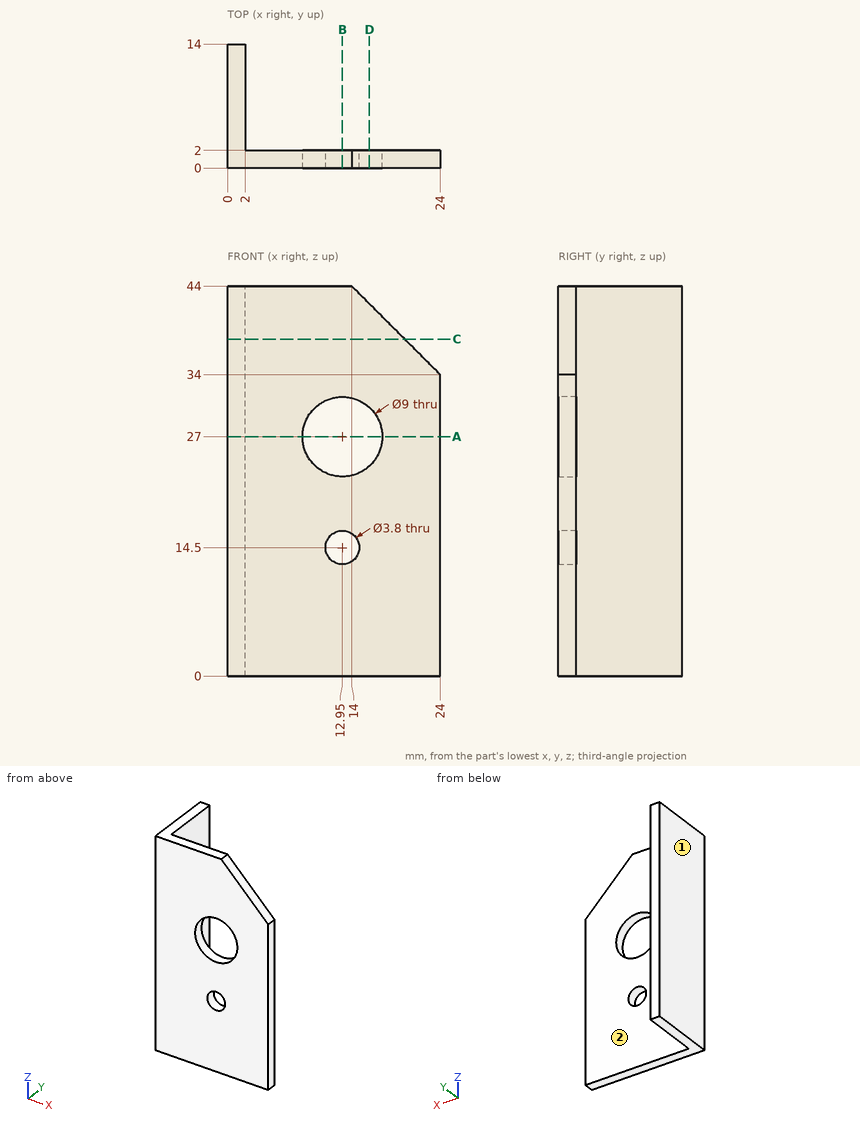
Part print with two shaded views. Sizes in mm from the minimum x, y, z corner. A direction names the side the tool comes from. Give positions to 0.01 mm unless a question says otherwise; leave off trailing zeros. Loops run counter-clockwise (first coordinate to the right, second up) from the corner with the lowest first, then second, coordinate; pieces in that order, holes last. Notation, with made-up numbers: (53.25, 75) - (79.25, 75) arc R6 cw to (79.25, 82) - close; hole circle Ø5 at (31.25, 22). An arc over 180 degrees is marked (long way). Put each result on its own line as item: value.
Q1. Slice it at D-D (x = 16). Give the cut face in (y, z).
Filled in:
outline: (0, 0) - (2, 0) - (2, 23.69) - (0, 23.69) - close; (0, 30.31) - (2, 30.31) - (2, 42) - (0, 42) - close
Q2. Probe line 1 along X through (y, z) = (1.3, 27); line 2 along Y through (x, z) = (21, 6); line 3 along X through (y, z) = (0.95, 14.5). List the from-to ranges inside material, lowest first.
Filled in:
line 1: x = 0 to 8.45, 17.45 to 24
line 2: y = 0 to 2
line 3: x = 0 to 11.05, 14.85 to 24
Q3. Slice it at C-C (z = 38). Give the cut face in (x, y).
Filled in:
outline: (0, 0) - (20, 0) - (20, 2) - (2, 2) - (2, 14) - (0, 14) - close
Q4. Flat gauge pins, fed straight in: pin 1 (5 mm diameter, centred on x = 12, z = 18, fed in from -Y); pin 2 (7 mm diameter, centred on x = 12.95, z = 27, fed in from -Y); pin 3 (5 mm diameter, centred on x = 12.95, z = 14.5, fed in from +Y). Where does each tip first touch, or does it go through?
Filled in:
pin 1: stops at y = 0
pin 2: passes through
pin 3: stops at y = 2
Q5. Slice it at A-A (z = 27). Give the cut face in (x, y), plus the area to 3 significant figures.
Filled in:
outline: (0, 0) - (8.45, 0) - (8.45, 2) - (2, 2) - (2, 14) - (0, 14) - close; (17.45, 0) - (24, 0) - (24, 2) - (17.45, 2) - close
area: 54.0 mm²
Q6. Slice it at B-B (x = 12.95). Give the cut face in (y, z), plus the area to 3 significant figures.
Filled in:
outline: (0, 0) - (2, 0) - (2, 12.6) - (0, 12.6) - close; (0, 16.4) - (2, 16.4) - (2, 22.5) - (0, 22.5) - close; (0, 31.5) - (2, 31.5) - (2, 44) - (0, 44) - close
area: 62.4 mm²
Q7. Tool access for the marked faces 1 and 2: list every direction of +Z, -Z, +X, -X, +Y, -Y with a clear straight run to the whole face (end or side of a thin tool).
Filled in:
face 1: +Z, -Z, -X, +Y, -Y
face 2: +Z, -Z, +X, +Y
